Verification items for the finished model (mm, model axes). Face numbers are marked on the shaded views. A direction names the side the tool comes from. Give positions to 0.01 mm unless a question says otherwise; leave off trailing zeros. Write each loop counter-clockwise with the first axis right and the second up, starting at its lowest first coordinate (ties: lowest second). Pieces come first, ordered by that corner, then holes. Notation, with made-up numbers: M -30.5,83 L -18.5,83 A20 ccw -18.5,121 Z; hole C 87.25,-30.75 d11. An arc over 180 degrees is marked long. Write item = value, one per line.
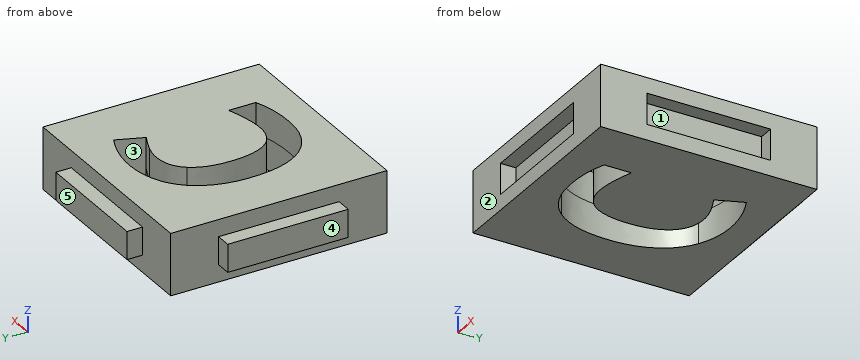
from build123d import *

# Parameters (mm, degrees)
F0_W     = 35.56
F0_H     = 35.56
F1_DEPTH = 5.08
F2_W     = 19.812
F2_H     = 4.572
F3_DEPTH = 2.54
F4_W     = 19.812
F4_H     = 4.572
F5_DEPTH = 2.54
F6_W     = 20.32
F6_H     = 5.08
F7_DEPTH = 2.54
F8_W     = 20.32
F8_H     = 5.08
F9_DEPTH = 2.54


with BuildPart() as f1:
    # F0 (on Top) → F1 (new body, symmetric)
    with BuildSketch(Plane.XY):
        Rectangle(F0_W, F0_H)
        with BuildLine():
            add(Edge.make_bspline(
                [(4.911328125, 7.9016710069), (3.4836805556, 8.4005208333), (2.1056423611, 8.4005208333)],
                knots=[0, 0, 0, 1, 1, 1], degree=2))
            add(Edge.make_bspline(
                [(2.1056423611, 8.4005208333), (-0.9095052083, 8.4005208333), (-2.5631510417, 6.1350260417)],
                knots=[0, 0, 0, 1, 1, 1], degree=2))
            add(Edge.make_bspline(
                [(-2.5631510417, 6.1350260417), (-4.216796875, 3.86953125), (-4.216796875, -0.1763888889)],
                knots=[0, 0, 0, 1, 1, 1], degree=2))
            add(Edge.make_bspline(
                [(-4.216796875, -0.1763888889), (-4.216796875, -8.5989583333), (2.1056423611, -8.5989583333)],
                knots=[0, 0, 0, 1, 1, 1], degree=2))
            add(Edge.make_bspline(
                [(2.1056423611, -8.5989583333), (4.7569878472, -8.5989583333), (8.5273003472, -7.2760416667)],
                knots=[0, 0, 0, 1, 1, 1], degree=2))
            Line((8.5273003472, -7.2760416667), (8.5273003472, -11.7519097222))
            add(Edge.make_bspline(
                [(8.5273003472, -11.7519097222), (5.4294704861, -13.047265625), (1.6040364583, -13.047265625)],
                knots=[0, 0, 0, 1, 1, 1], degree=2))
            add(Edge.make_bspline(
                [(1.6040364583, -13.047265625), (-3.8915798611, -13.047265625), (-6.8019965278, -9.7124131944)],
                knots=[0, 0, 0, 1, 1, 1], degree=2))
            add(Edge.make_bspline(
                [(-6.8019965278, -9.7124131944), (-9.7124131944, -6.3775607639), (-9.7124131944, -0.1433159722)],
                knots=[0, 0, 0, 1, 1, 1], degree=2))
            add(Edge.make_bspline(
                [(-9.7124131944, -0.1433159722), (-9.7124131944, 3.7868489583), (-8.2820095486, 6.7413628472)],
                knots=[0, 0, 0, 1, 1, 1], degree=2))
            add(Edge.make_bspline(
                [(-8.2820095486, 6.7413628472), (-6.8516059028, 9.6958767361), (-4.1726996528, 11.2695963542)],
                knots=[0, 0, 0, 1, 1, 1], degree=2))
            add(Edge.make_bspline(
                [(-4.1726996528, 11.2695963542), (-1.4937934028, 12.8433159722), (2.1056423611, 12.8433159722)],
                knots=[0, 0, 0, 1, 1, 1], degree=2))
            add(Edge.make_bspline(
                [(2.1056423611, 12.8433159722), (5.7712239583, 12.8433159722), (9.475390625, 11.0739149306)],
                knots=[0, 0, 0, 1, 1, 1], degree=2))
            Line((9.475390625, 11.0739149306), (7.7555989583, 6.7303385417))
            add(Edge.make_bspline(
                [(7.7555989583, 6.7303385417), (6.3389756944, 7.4028211806), (4.911328125, 7.9016710069)],
                knots=[0, 0, 0, 1, 1, 1], degree=2))
        make_face(mode=Mode.SUBTRACT)
    extrude(amount=F1_DEPTH, both=True)

    # F2 (on face) → F3 (join)
    with BuildSketch(Plane(origin=(0, 17.78, 0), x_dir=(-1, 0, 0), z_dir=(0, 1, 0))):
        Rectangle(F2_W, F2_H)
    extrude(amount=F3_DEPTH)

    # F4 (on face) → F5 (join)
    with BuildSketch(Plane(origin=(-17.78, 0, 0), x_dir=(0, -1, 0), z_dir=(-1, 0, 0))):
        Rectangle(F4_W, F4_H)
    extrude(amount=F5_DEPTH)

    # F6 (on face) → F7 (cut)
    with BuildSketch(Plane.XZ.offset(17.78)):
        Rectangle(F6_W, F6_H)
    extrude(amount=-F7_DEPTH, mode=Mode.SUBTRACT)

    # F8 (on face) → F9 (cut)
    with BuildSketch(Plane.YZ.offset(17.78)):
        Rectangle(F8_W, F8_H)
    extrude(amount=-F9_DEPTH, mode=Mode.SUBTRACT)


solid = f1.part
1) Depth check by flat-ended pin: P1, Ø1.5, axis at y = -13, z = -0.5, coming from the -X side; P2, Ø0.8, axis at x = 16.5, z = -0.5, coming from the +Y side; P3, Ø0.8, axis at x = -19, y = 1.5, coming from the -Z side. Enter the tip coordinate at first touch or a pass-through.
From the geometry:
P1 = -17.78
P2 = 17.78
P3 = -2.29
2) Draft check along X on the marked faces 3, 4 and 5. Enter one of: +X half, -X half, draft (parallel to the pull), parting line (faces both ways), or undercut.
From the geometry:
face_3 = undercut
face_4 = -X half
face_5 = draft
3) Tool access check on the marked faces 1 and 2. Record the directions out of +Z, -Z, +X, -X, +Y, -Y that give a thin tool (end or side, any length) a straight path to the whole face; none if there is none.
From the geometry:
face_1 = +X
face_2 = +Z, -Z, +X, -X, -Y
4) Cross-section at A-A on y = 15. Record the boundary of the cut face in (x, z), plus the area to 3 significant figures.
From the geometry:
outline = M -17.78,-5.08 L 17.78,-5.08 L 17.78,5.08 L -17.78,5.08 Z
area = 361 mm^2
5) Material ranges on probe 1 along Y at (x, z) = (0, 1); probe 2 along Y at (x, z) = (0.5, 3.75); probe 3 along X at (y, z) = (15.5, 3.75), recorded low to high. Write a range as from..to.
From the geometry:
probe_1 = -15.24..-12.97, -8.32..8.07, 12.7..20.32
probe_2 = -17.78..-13.01, -8.44..8.22, 12.76..17.78
probe_3 = -17.78..17.78
